Autodesk Inventor part; units mm, degrees
ref_plane "YZ Plane" through (0, 0, 0) normal (1, 0, 0) x (0, 1, 0)
ref_plane "XZ Plane" through (0, 0, 0) normal (0, 1, 0) x (-1, 0, 0)
ref_plane "XY Plane" through (0, 0, 0) normal (0, 0, 1) x (1, 0, 0)
sketch "Schizzo1" plane through (0, 0, 0) normal (0, 0, 1) x (1, 0, 0)
  line L0 (-5, 60) -> (5, 60)
  line L1 (5, 60) -> (5, -60)
  line L2 (5, -60) -> (-5, -60)
  line L3 (-5, -60) -> (-5, 60)
  line L4 (-5, 60) -> (5, -60) construction
  line L5 (5, 60) -> (-5, -60) construction
  line L6 (-5, 40) -> (5, 40)
  line L7 (5, 40) -> (5, -40)
  line L8 (5, -40) -> (-5, -40)
  line L9 (-5, -40) -> (-5, 40)
  line L10 (-5, 40) -> (5, -40) construction
  line L11 (5, 40) -> (-5, -40) construction
  line L12 (0, 0) -> (121.0573, 0)
  line L13 (0, 0) -> (0, 96.1234)
  dimension "d0" = 120
  dimension "d1" = 10
  dimension "d2" = 80
extrude "Estrusione1" add sketch "Schizzo1" along normal blind 100
extrude "Estrusione2" add sketch "Schizzo1" against normal blind 100 contours L6 L13 L12 L1 L8 L3 | L6 L1 L12 L13
fillet "Raccordo1" radius 4 2 edges at (0, 40, 0) (0, -40, 0)
properties part number "05-23-2023 FEM"
The listing builds one solid part. Answer for the finished solid, in the listing's coordinates (mm). A direction names the side the tool comes from. Round coordinates to 2 decimals unless told otherwise and drop trailing zeros. Loops run counter-clockwise (first coordinate to the right, second up) from the corner with the lowest first, then second, coordinate; pieces in that order, holes last. Notation, with made-up numbers: (2, 41.25) - (31, 41.25) arc R19 ccw to (31, 59.25) - close; hole circle Ø10 at (28, 80.5). An arc over 180 degrees is marked (long way). Return JSON: item names as keys, results as strings. Group by question number.
1. Each of these flat-tipped pins is pushed along its axis until it touches: P1, Ø5, axis at x = 0, z = -47, coming from the +Y side; P2, Ø3, axis at x = -1.5, y = 50.5, coming from the -Z side; P3, Ø3, axis at x = -1.5, z = -34.5, coming from the -Y side. Where does it stop, or does it pass through?
2. The part is cut by section A-A on x = 2.75. Determine the outline of the cut face in (y, z).
3. The part is cut by section B-B on y = -48. Determine the outline of the cut face in (x, z), then the cut area to 3 significant figures.
4. The part is cut by section C-C on z = -77. Determine the outline of the cut face in (x, y), then the cut area to 3 significant figures.
5. Consider probe 1 along Y at (x, z) = (-3, -59.5); probe 2 along Z at (x, y) = (-2, 48); probe 3 along Z at (x, y) = (-1, -42). Determine where each line is inside the solid, lowest interval first.
6. Which of the six approach directions +Z, -Z, +X, -X, +Y, -Y give full straight-line access (tool end or side, diameter ignored) to faces 1 (the flat face through (0, -40, -51)), 2 (the flat face through (0, 1, -100)), 3 (the flat face through (0, 52, 0))?
Resolved:
{
 "1": {"P1": "stops at y = 40", "P2": "stops at z = 0", "P3": "stops at y = -40"},
 "2": {"outline": "(-60, 0) - (-44, 0) arc R4 cw to (-40, -4) - (-40, -100) - (40, -100) - (40, -4) arc R4 cw to (44, 0) - (60, 0) - (60, 100) - (-60, 100) - close"},
 "3": {"outline": "(-5, 0) - (5, 0) - (5, 100) - (-5, 100) - close", "area": "1,000 mm²"},
 "4": {"outline": "(-5, -40) - (5, -40) - (5, 40) - (-5, 40) - close", "area": "800 mm²"},
 "5": {"probe 1": "y = -40 to 40", "probe 2": "z = 0 to 100", "probe 3": "z = -0.54 to 100"},
 "6": {"face 1": "-Z, +X, -X, -Y", "face 2": "-Z, +X, -X, +Y, -Y", "face 3": "-Z, +X, -X, +Y"}
}
